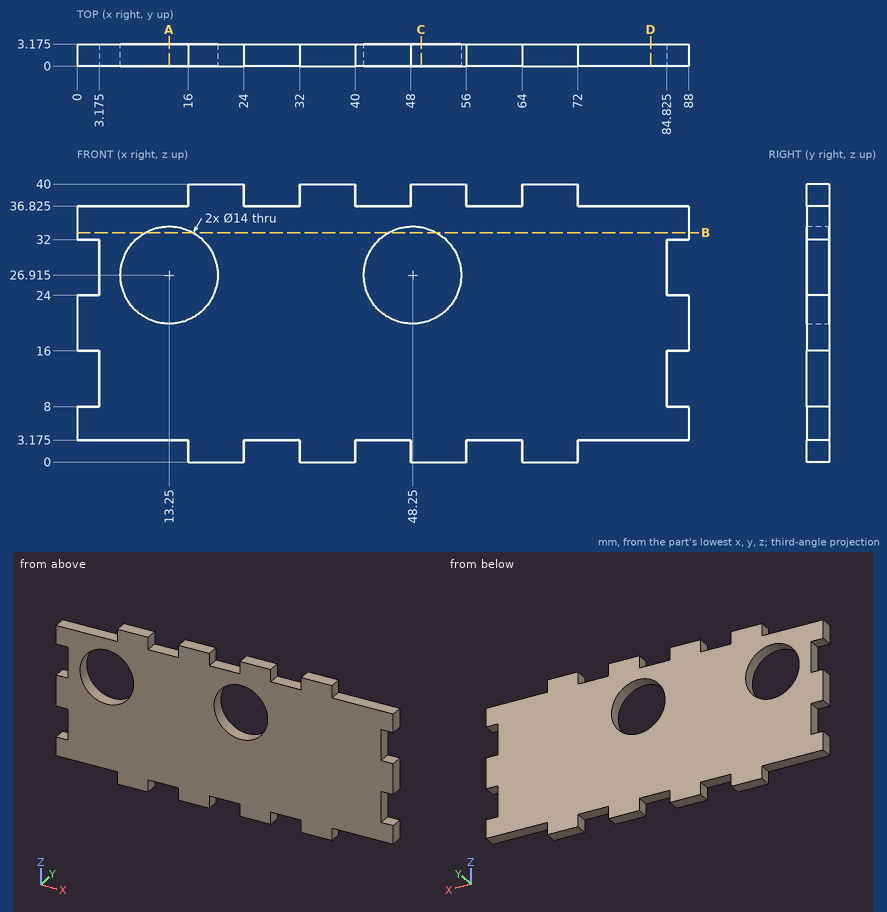
Job drawing, mm, ordinate dimensions from the low corner. One solid piece. Give positions to 0.01 mm unless a question says otherwise; leave off trailing zeros. Loops run counter-clockwise (first coordinate to the right, second up) from the corner with the lowest first, then second, coordinate; pieces in that order, holes last. Notation, with made-up numbers: (25.25, 43.25) -> (81.25, 43.25) arc R21 cw to (81.25, 77.25) -> close; hole circle Ø6 at (85.5, -2.75). An arc over 180 degrees is marked (long way). Use a Markdown table: item, result. Add a question column.
(1) Wall check: line 1 along X through (y, z) = (2.1, 3); line 2 along X through (y, z) = (0.4, 26) (3 decimals); line 3 along Z through (x, y) = (13.25, 2.5) (3 decimals). Give the ranges that are in metal, low to high.
(2) Slice it at D-D on x = 82.5. List the corners of the cut face in (y, z) (3 decimals), and give its area (3 significant figures).
(3) Slice it at C-C on x = 49.5. List the corners of the cut face in (y, z) (3 decimals), and give its area (3 significant figures).
(4) Slice it at A-A on x = 13.25. List the corners of the cut face in (y, z) (3 decimals), and give its area (3 significant figures).
(5) Drop flat-ended pins along their axis: pin 1 Ø1.6 at (x, y) = (2.5, 2) entering from -Z (3 decimals); pin 2 Ø1 at (y, z) = (1, 13.5) entering from +X (3 decimals); pin 3 Ø1 at (y, z) = (2, 2) entering from -X; pin 4 Ø6 at (x, z) = (48.5, 6) entering from -Y. Give the stop position or say it passes through.
(6) Slice it at B-B on z = 33. List the corners of the cut face in (x, y) (3 decimals).
Filled sheet:
| question | item | result |
|---|---|---|
| 1 | line 1 | 16 to 24, 32 to 40, 48 to 56, 64 to 72 |
| 1 | line 2 | 3.175 to 6.31, 20.19 to 41.31, 55.19 to 84.825 |
| 1 | line 3 | 3.175 to 19.915, 33.915 to 36.825 |
| 2 | outline | (0, 3.175) -> (3.175, 3.175) -> (3.175, 36.825) -> (0, 36.825) -> close |
| 2 | area | 107 mm2 |
| 3 | outline | (0, 0) -> (3.175, 0) -> (3.175, 20.028) -> (0, 20.028) -> close; (0, 33.802) -> (3.175, 33.802) -> (3.175, 40) -> (0, 40) -> close |
| 3 | area | 83.3 mm2 |
| 4 | outline | (0, 3.175) -> (3.175, 3.175) -> (3.175, 19.915) -> (0, 19.915) -> close; (0, 33.915) -> (3.175, 33.915) -> (3.175, 36.825) -> (0, 36.825) -> close |
| 4 | area | 62.4 mm2 |
| 5 | pin 1 | z = 3.175 |
| 5 | pin 2 | x = 84.825 |
| 5 | pin 3 | x = 16 |
| 5 | pin 4 | y = 0 |
| 6 | outline | (0, 0) -> (9.79, 0) -> (9.79, 3.175) -> (0, 3.175) -> close; (16.71, 0) -> (44.79, 0) -> (44.79, 3.175) -> (16.71, 3.175) -> close; (51.71, 0) -> (88, 0) -> (88, 3.175) -> (51.71, 3.175) -> close |
